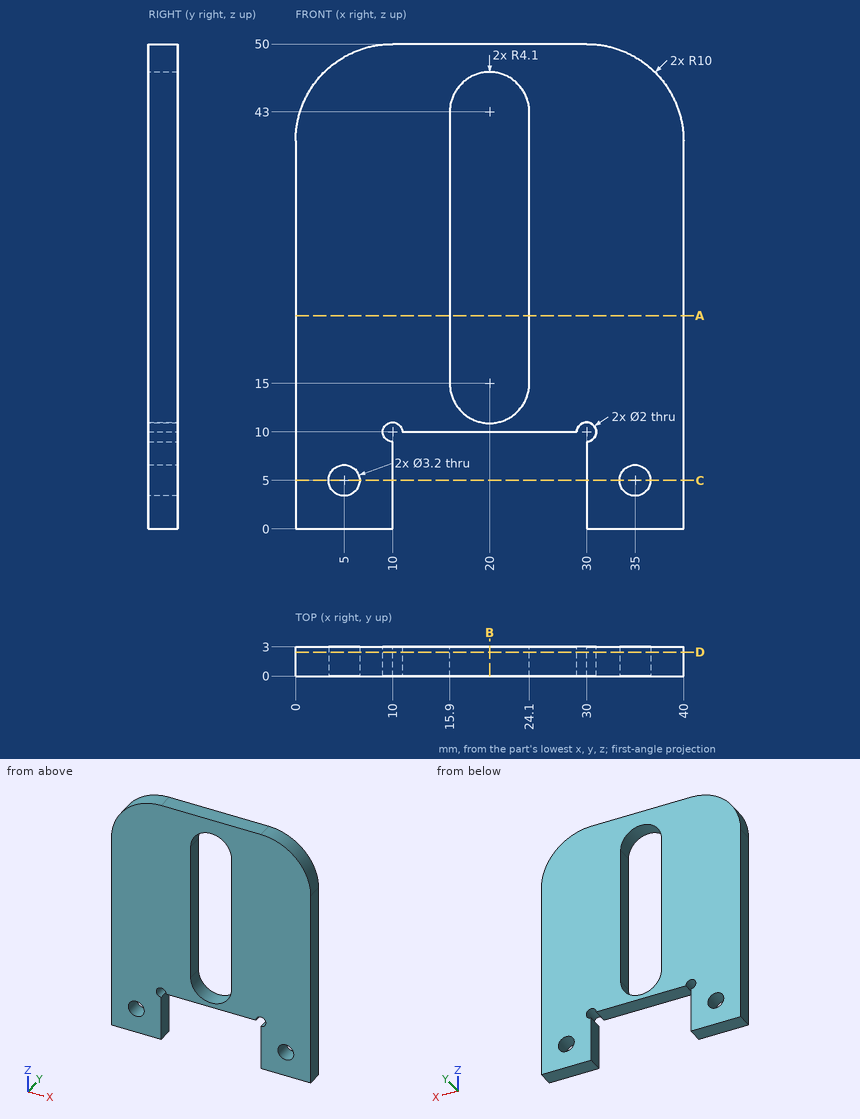
Can you work these out from the drawing? Everything is in mm from the part's minimum corner. Coordinates: 2 decimals unless noted, no trailing zeros. Order: outer loops, then holes, each group sorted by start corner. A loop starts at its lowest first (then second) coordinate and runs counter-clockwise, first axis right, second up. Notation, with made-up numbers: M 24,-12 L 73,-12 A12 cw 73,10 Z; hole C -17.5,68 d11. An arc over 180 degrees is marked long. Answer as CSV lines item,"result". Start each with the question number.
1. I want a section at B-B, the plane x = 20. Write out the boundary of the cut face in (y, z).
2. I want a section at A-A, the plane z = 22. Write out the boundary of the cut face in (x, y), and give its area (3 significant figures).
3. I want a section at D-D, the plane y = 2.45. Write out the boundary of the cut face in (x, z).
4. For pin 1 (1.6 mm diameter, centred on x = 30, z = 10, fed in from +Y); pin 2 (1 mm diameter, centred on y = 2, z = 41, fed in from -X), each with a flat end and sliding along its axis, tell me the tip position at first contact or that it passes through.
5. I need wall thicknesses on line 1 (X direction, y = 1.4, z = 5); line 2 (X direction, y = 1.55, z = 23.5); line 3 (Z direction, x = 22.5, y = 2). Which ranges of each line are inside material? Lowest first, please. Write a range as [from, to].
6. I want a section at C-C, the plane z = 5. Write out the boundary of the cut face in (x, y).
Recorded:
1,outline,"M 0,10 L 3,10 L 3,10.9 L 0,10.9 Z; M 0,47.1 L 3,47.1 L 3,50 L 0,50 Z"
2,outline,"M 0,0 L 15.9,0 L 15.9,3 L 0,3 Z; M 24.1,0 L 40,0 L 40,3 L 24.1,3 Z"
2,area,"95.4 mm2"
3,outline,"M 0,0 L 10,0 L 10,9 A1 cw long 11,10 L 29,10 A1 cw long 30,9 L 30,0 L 40,0 L 40,40 A10 ccw 30,50 L 10,50 A10 ccw 0,40 Z; hole C 5,5 d3.2; hole M 15.9,15 A4.1 ccw 24.1,15 L 24.1,43 A4.1 ccw 15.9,43 Z; hole C 35,5 d3.2"
4,pin 1,"passes through"
4,pin 2,"stops at x = 0.01"
5,line 1,"x = [0, 3.4], [6.6, 10], [30, 33.4], [36.6, 40]"
5,line 2,"x = [0, 15.9], [24.1, 40]"
5,line 3,"z = [10, 11.75], [46.25, 50]"
6,outline,"M 0,0 L 3.4,0 L 3.4,3 L 0,3 Z; M 6.6,0 L 10,0 L 10,3 L 6.6,3 Z; M 30,0 L 33.4,0 L 33.4,3 L 30,3 Z; M 36.6,0 L 40,0 L 40,3 L 36.6,3 Z"
